Here's the drawing with two shaded views (mm, measured from the low corner). I have some questions. A direction names the side the tool comes from. Give positions to 0.01 mm unless a question says otherwise; leave off trailing zeros. Write each loop counter-clockwise with the first axis right and the second up, starting at its lowest first coordinate (ties: lowest second). Pieces come first, ordered by that corner, then holes.
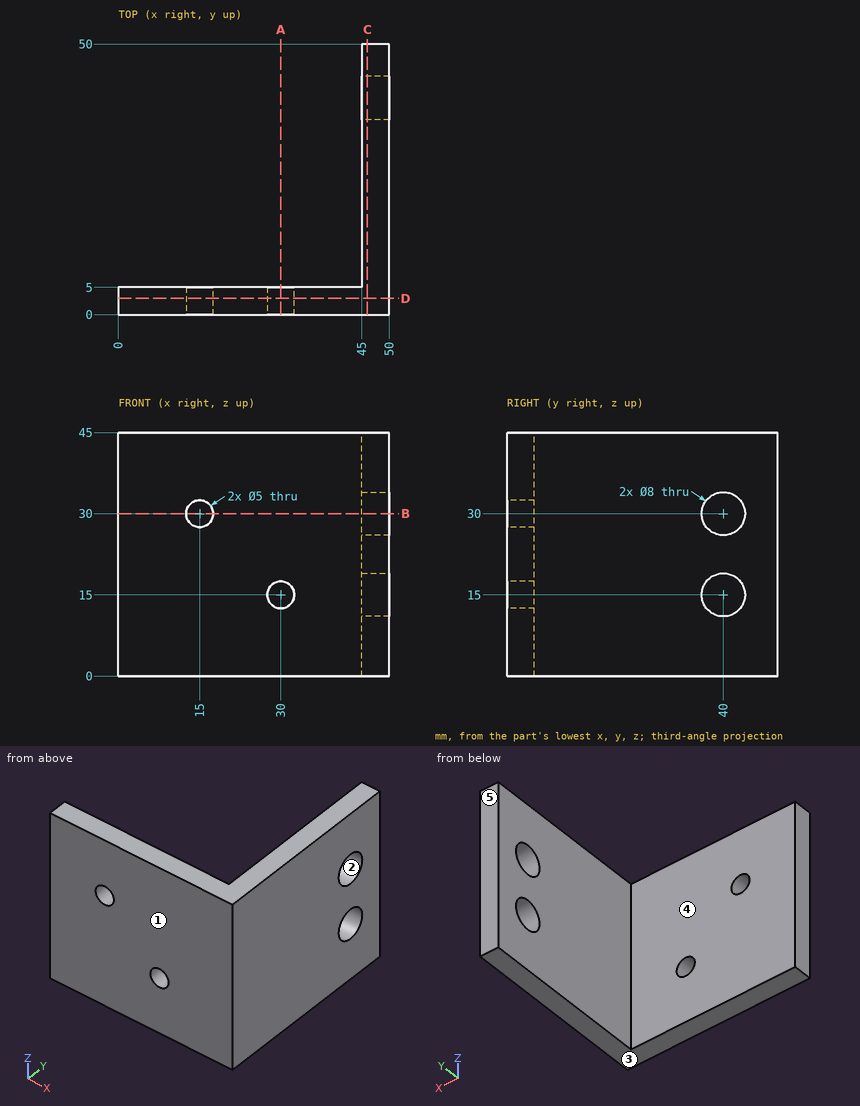
1) For the marked faces 4 and 5, which set-ups out of +Z, -Z, +X, -X, +Y, -Y let a thin tool reach every point of the face, with its end or its side?
Values follow:
face 4: +Z, -Z, -X, +Y
face 5: +Z, -Z, +X, -X, +Y
2) Suppose I cut it at A-A on x = 30. Write out the boundary of the cut face in (y, z).
Values follow:
outline: (0, 0) - (5, 0) - (5, 12.5) - (0, 12.5) - close; (0, 17.5) - (5, 17.5) - (5, 45) - (0, 45) - close
3) Suppose I cut it at B-B on z = 30. Write out the boundary of the cut face in (x, y).
Values follow:
outline: (0, 0) - (12.5, 0) - (12.5, 5) - (0, 5) - close; (17.5, 0) - (50, 0) - (50, 36) - (45, 36) - (45, 5) - (17.5, 5) - close; (45, 44) - (50, 44) - (50, 50) - (45, 50) - close
4) Suppose I cut it at D-D on y = 3. Write out the boundary of the cut face in (x, z), plus the area to 3 significant figures.
Values follow:
outline: (0, 0) - (50, 0) - (50, 45) - (0, 45) - close; hole circle Ø5 at (15, 30); hole circle Ø5 at (30, 15)
area: 2,210 mm2
5) Suppose I cut it at C-C on x = 46. Write out the boundary of the cut face in (y, z).
Values follow:
outline: (0, 0) - (50, 0) - (50, 45) - (0, 45) - close; hole circle Ø8 at (40, 15); hole circle Ø8 at (40, 30)
6) If we mould it in two halves opening along Z, with no side actions, what happens to the marked faces 1, 2 and 3? For each: +Z half, -Z half, draft (parallel to the pull), parting line (faces both ways), or undercut.
Values follow:
face 1: draft
face 2: undercut
face 3: -Z half
7) Please list where these lines run through material, in increasing order: L1, parallel to Y at x = 48.5, z = 30; L2, parallel to Z at x = 30, y = 2.6; L3, parallel to X at y = 2, z = 30.
Values follow:
L1: y = 0 to 36, 44 to 50
L2: z = 0 to 12.5, 17.5 to 45
L3: x = 0 to 12.5, 17.5 to 50
8) For pin 1 Ø13.5 at (y, z) = (27.5, 19) entering from -X; pin 2 Ø4 at (x, z) = (30, 15) entering from -Y; pin 3 Ø1.5 at (x, z) = (5.5, 15.5) entering from +Y, each with a flat end and sliding along its axis, tell me the tip position at first contact or that it passes through.
Values follow:
pin 1: stops at x = 45
pin 2: passes through
pin 3: stops at y = 5
